```python
from build123d import *

# Parameters (mm, degrees)
F0_R     = 8.0772
F1_DEPTH = 50.48541
F2_R     = 12.7227956512
F3_DEPTH = 25.4
F5_DEPTH = 25.4


# Not quite as in the source:
# - a fillet or chamfer that OpenCascade refuses, or shapes differently, is made with other operations: its cross-section is extruded or revolved along the edge and cut away or added


with BuildPart() as f1:
    # F0 (on Top) → F1 (new body)
    with BuildSketch(Plane.XY):
        Circle(F0_R)
    extrude(amount=F1_DEPTH)

    # F2 (on face) → F3 (join)
    with BuildSketch(Plane.XY.offset(50.48541)):
        Circle(F2_R)
    extrude(amount=F3_DEPTH)

    # F4 (on face) → F5 (cut)
    with BuildSketch(Plane.XY.offset(75.88541)):
        with BuildLine():
            Line((9.0839408688, -8.9079485558), (-9.0839408688, -8.9079485558))
            ThreePointArc((-9.0839408688, -8.9079485558), (0, -12.7227956512), (9.0839408688, -8.9079485558))
        make_face()
    extrude(amount=-F5_DEPTH, mode=Mode.SUBTRACT)

    # F6: chamfer of 1.27 on 2 edges, made by hand


with BuildPart() as f6_tool2:
    # F6_s3 → F6_t4 (revolve)
    with BuildSketch(Plane.XZ):
        Polygon((9.3472, 50.48541), (8.0772, 49.21541), (8.0772, 50.48541), align=None)
    revolve(axis=Axis((0, 0, 50.48541), (0, 0, 1)))

    split(bisect_by=Plane.XZ.offset(8.9079485558), keep=Keep.BOTTOM)


with BuildPart() as f1_1:
    add(f1.part)

    # F6_t1: union F6_tool2
    add(f6_tool2.part)

    # F6_s6 → F6_t7 (revolve, cut)
    with BuildSketch(Plane.XZ):
        Polygon((8.0772, 1.27), (6.8072, 0), (8.0772, 0), align=None)
    revolve(axis=Axis((0, 0, 0), (0, 0, 1)), mode=Mode.SUBTRACT)


solid = f1_1.part
```
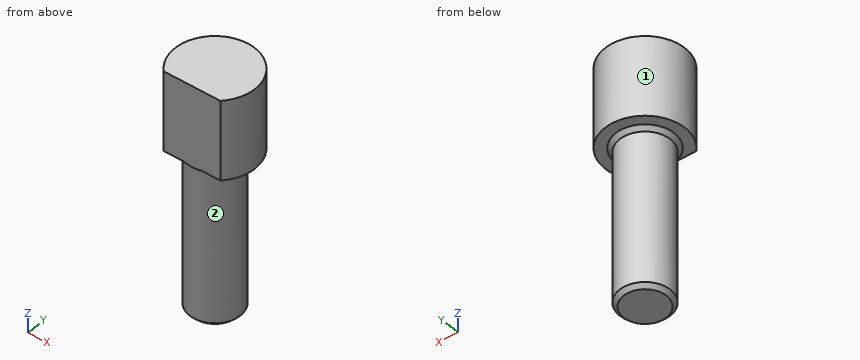
Work out the finished part from the listing and answer in its coordinate system (mm). Face numbers are marked on the shaded views. A direction names the side the tool comes from. Coordinates: 2 decimals unless noted, no trailing zeros. Write each loop counter-clockwise with the first axis right and the second up, starting at its lowest first coordinate (ties: lowest second). Pieces come first, ordered by that corner, then holes.
Q1. A cutting plane is placed at D-D, the plane z = 23.5. Give the vertices of the cut face in (x, y).
Q2. A cutting plane is placed at B-B, the plane y = 0. Give the vertices of the cut face in (x, z), then the cut area to 3 significant figures.
Q3. Each of these flat-tipped pins is pushed along its axis until it touches: pin 1 Ø1.5 at (y, z) = (6.5, 57) entering from +X; pin 2 Ø1.5 at (y, z) = (0, 24) entering from -X; pin 3 Ø2 at (y, z) = (7, 21.5) entering from +X. Where does it stop, or does it pass through?
Q4. Find the intervals of material crossed by line 1 (Z direction, x = 6.5, y = 7.5); line 2 (X direction, y = 10.5, z = 53); line 3 (Y direction, x = -11, z = 71.5), in increasing order.
Q5. Which of the six approach directions +Z, -Z, +X, -X, +Y, -Y give full straight-line access (tool end or side, diameter ignored) to the marked faces 1 and 2?
Q6. A cutting plane is placed at A-A, the plane x = 0. Give the vertices of the cut face in (y, z).
Q7. A cutting plane is placed at C-C, the plane z = 57. Give the vertices of the cut face in (x, y).
Findings below:
1. outline: circle Ø16.15 at (0, 0)
2. outline: (-12.72, 50.49) - (-9.35, 50.49) - (-8.08, 49.22) - (-8.08, 1.27) - (-6.81, 0) - (6.81, 0) - (8.08, 1.27) - (8.08, 49.22) - (9.35, 50.49) - (12.72, 50.49) - (12.72, 75.89) - (-12.72, 75.89) - close
2. area: 1,460 mm2
3. pin 1: stops at x = 11.35
3. pin 2: stops at x = -8.08
3. pin 3: stops at x = 5.41
4. line 1: z = 50.49 to 75.89
4. line 2: x = -7.18 to 7.18
4. line 3: y = -6.39 to 6.39
5. face 1: +Z, -Z
5. face 2: -Z
6. outline: (-8.91, 50.05) - (-8.08, 49.22) - (-8.08, 1.27) - (-6.81, 0) - (6.81, 0) - (8.08, 1.27) - (8.08, 49.22) - (9.35, 50.49) - (12.72, 50.49) - (12.72, 75.89) - (-8.91, 75.89) - close
7. outline: (-9.08, -8.91) - (9.08, -8.91) arc R12.72 ccw (long way) to start
